CAD build for the part. Positions are in the model's coordinates, mm. Face numbers are marked on the shaded views. A direction names the side the tool comes from. Coordinates: 2 decimals unless noted, no trailing zeros. Write each loop counter-clockwise with the first axis right and the second up, starting at its lowest first coordinate (ties: lowest second). Pieces come first, ordered by that corner, then holes. Notation, with made-up numbers: (5.5, -17) -> (61.5, -17) arc R22 ccw to (61.5, 15) -> close; hole circle Ø8 at (-37, -9). An arc over 180 degrees is marked (long way). Answer as CSV lines item,"result".
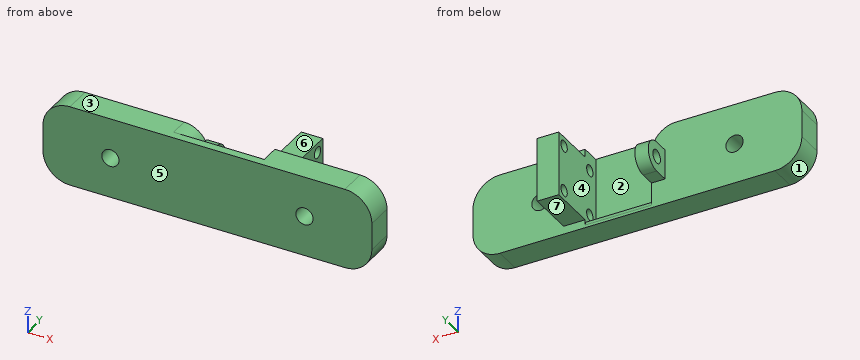
```python
from build123d import *

# Parameters (mm, degrees)
SKETCH1_W           = 122
SKETCH1_H           = 30
BOSS_EXTRUDE1_DEPTH = 10
SKETCH2_W           = 24
SKETCH2_H           = 17.447802
BOSS_EXTRUDE2_DEPTH = 8
SKETCH3_R           = 2.475
BOSS_EXTRUDE3_DEPTH = 5
SKETCH4_W           = 24.63
SKETCH4_H           = 27
CUT_EXTRUDE1_DEPTH  = 7
FILLET1_R           = 10
SKETCH7_R           = 3.2
CUT_EXTRUDE2_DEPTH  = 66.195289666
BOSS_EXTRUDE5_START = 1
SKETCH8_R           = 3.1
SKETCH8_R_2         = 2.475
BOSS_EXTRUDE5_DEPTH = 1
FILLET2_R           = 9
FILLET3_R           = 2
SKETCH9_R           = 2.1
CUT_EXTRUDE3_DEPTH  = 8


with BuildPart() as part:
    # Sketch1 → Boss-Extrude1 (new body)
    with BuildSketch(Plane(origin=(0, 0, 0), x_dir=(1, 0, 0), z_dir=(0, 1, 0))):
        Rectangle(SKETCH1_W, SKETCH1_H)
    extrude(amount=BOSS_EXTRUDE1_DEPTH)

    # Sketch2 → Boss-Extrude2 (add)
    with BuildSketch(Plane(origin=(19.38, 0, 0), x_dir=(0, 0, -1), z_dir=(1, 0, 0))):
        with Locations((0, 18.723901)):
            Rectangle(SKETCH2_W, SKETCH2_H)
    extrude(amount=BOSS_EXTRUDE2_DEPTH)

    # Sketch3 → Boss-Extrude3 (add)
    with BuildSketch(Plane(origin=(-5.25, 0, 0), x_dir=(0, 0, -1), z_dir=(1, 0, 0))):
        with BuildLine():
            Line((-5.552198, 15.552198), (-5.552198, 10))
            Line((-5.552198, 10), (5.552198, 10))
            Line((5.552198, 10), (5.552198, 15.552198))
            ThreePointArc((5.552198, 15.552198), (0, 21.104396), (-5.552198, 15.552198))
        make_face()
        with Locations((0, 15.552198)):
            Circle(SKETCH3_R, mode=Mode.SUBTRACT)
    extrude(amount=-BOSS_EXTRUDE3_DEPTH)

    # Sketch4 → Cut-Extrude1 (cut)
    with BuildSketch(Plane(origin=(0, 10, 0), x_dir=(1, 0, 0), z_dir=(0, 1, 0))):
        with Locations((7.065, -1.5)):
            Rectangle(SKETCH4_W, SKETCH4_H)
    extrude(amount=-CUT_EXTRUDE1_DEPTH, mode=Mode.SUBTRACT)

    # Fillet1
    fillet1_edges = [part.edges().sort_by_distance(p)[0] for p in [
        (61, 5, 15),
        (-61, 5, 15),
        (-61, 5, -15),
        (61, 5, -15),
    ]]
    fillet(fillet1_edges, radius=FILLET1_R)

    # Sketch7 → Cut-Extrude2 (cut, through all)
    with BuildSketch(Plane(origin=(0, 10, 0), x_dir=(1, 0, 0), z_dir=(0, 1, 0))):
        with Locations(Location((-36, 0, 0), (0, 0, 270))):
            Circle(SKETCH7_R)
        with Locations(Location((36, 0, 0), (0, 0, 90))):
            Circle(SKETCH7_R)
    extrude(amount=-CUT_EXTRUDE2_DEPTH, mode=Mode.SUBTRACT)

    # Sketch8 → Boss-Extrude5 (add)
    with BuildSketch(Plane(origin=(-5.25, 0, 0), x_dir=(0, 0, -1), z_dir=(1, 0, 0)).offset(BOSS_EXTRUDE5_START)):
        with Locations((0, 15.552198)):
            Circle(SKETCH8_R)
        with Locations((0, 15.552198)):
            Circle(SKETCH8_R_2, mode=Mode.SUBTRACT)
    extrude(amount=-BOSS_EXTRUDE5_DEPTH)

    # Fillet2
    fillet2_edges = [part.edges().sort_by_distance(p)[0] for p in [
        (-5.25, 6.5, 15),
    ]]
    fillet(fillet2_edges, radius=FILLET2_R)

    # Fillet3
    fillet3_edges = [part.edges().sort_by_distance(p)[0] for p in [
        (7.065, 10, -12),
    ]]
    fillet(fillet3_edges, radius=FILLET3_R)

    # Sketch9 → Cut-Extrude3 (cut)
    with BuildSketch(Plane.ZY.offset(-19.38)):
        with Locations((8.5, 23.947802)):
            Circle(SKETCH9_R)
        with Locations((8.5, 6.947802)):
            Circle(SKETCH9_R)
        with Locations((-8.5, 6.947802)):
            Circle(SKETCH9_R)
        with Locations((-8.5, 23.947802)):
            Circle(SKETCH9_R)
    extrude(amount=-CUT_EXTRUDE3_DEPTH, mode=Mode.SUBTRACT)


solid = part.part
```
Item 1: Two-plate mould, pull along X, no slides. Class the marked faces 1, 2, 3 and 4: pulls with the +X half, pulls with the -X half, needs draft (parallel to the pull), parting line crosses it, or undercut.
Answer below:
face 1,"pulls with the -X half"
face 2,"undercut"
face 3,"needs draft"
face 4,"undercut"
Item 2: Saw through at C-C on x = 18. Give the cut face in (y, z).
Answer below:
outline,"(0, -15) -> (10, -15) -> (10, -14) arc R2 ccw to (8, -12) -> (3, -12) -> (3, 15) -> (0, 15) -> close"
Item 3: Saw through at D-D on z = -8.5. Give the cut face in (x, y), and give its area (3 significant figures).
Answer below:
outline,"(-60.37, 0) -> (60.37, 0) -> (60.37, 10) -> (27.38, 10) -> (27.38, 21.85) -> (19.38, 21.85) -> (19.38, 9.05) -> (27.38, 9.05) -> (27.38, 4.85) -> (19.38, 4.85) -> (19.38, 3) -> (-5.25, 3) -> (-5.25, 10) -> (-60.37, 10) -> close; (19.38, 26.05) -> (27.38, 26.05) -> (27.38, 27.45) -> (19.38, 27.45) -> close"
area,"1,110 mm2"
Item 4: Saw through at B-B on z = 8.5. Give the cut face in (x, y).
Answer below:
outline,"(-60.37, 0) -> (60.37, 0) -> (60.37, 10) -> (27.38, 10) -> (27.38, 21.85) -> (19.38, 21.85) -> (19.38, 9.05) -> (27.38, 9.05) -> (27.38, 4.85) -> (19.38, 4.85) -> (19.38, 3) -> (-5.6, 3) -> (-5.6, 10) -> (-60.37, 10) -> close; (19.38, 26.05) -> (27.38, 26.05) -> (27.38, 27.45) -> (19.38, 27.45) -> close"
Item 5: Flat gauge pins, fed straight in: pin 1 (5.5 mm diameter, centred on x = -8, y = 12, fed in from +Z); pin 2 (4 mm diameter, centred on y = 6.95, z = -8.5, fed in from +X); pin 3 (4.5 mm diameter, centred on y = 15.55, z = 0, fed in from -X). Where does each tip first touch, or does it go through?
Answer below:
pin 1,"stops at z = 13.87"
pin 2,"stops at x = 60.89"
pin 3,"stops at x = 19.38"
Item 6: Wall check: line 1 (X direction, y = 6.75, z = 0); line 2 (X direction, y = 13.5, z = 4); line 3 (X direction, y = 18.5, z = 0.5). Give the ranges that are in metal, low to high. Write a range as from..to.
Answer below:
line 1,"x = -61..-39.2, -32.8..-5.25, 19.38..32.8, 39.2..61"
line 2,"x = -10.25..-5.25, 19.38..27.38"
line 3,"x = -10.25..-4.25, 19.38..27.38"
Item 7: Saw through at A-A on x = -36. Give the cut face in (y, z).
Answer below:
outline,"(0, -15) -> (10, -15) -> (10, -3.2) -> (0, -3.2) -> close; (0, 3.2) -> (10, 3.2) -> (10, 15) -> (0, 15) -> close"
Item 8: 3-axis set-ups, long thin cutter, end or side, ignore diameter. For the marked faces 5, 6 and 7: which of +Z, -Z, +X, -X, +Y, -Y reach the whole face in a straight line?
Answer below:
face 5,"+Z, -Z, +X, -X, -Y"
face 6,"+Z, +X, -X, +Y"
face 7,"-Z, +X, -X, +Y"
